```python
from build123d import *

# Parameters (mm, degrees)
BASE_DEPTH              = 5
BASE_DEPTH_BACK         = 5
ESQUISSE1_R             = 2
ESQUISSE2_W             = 77.5
ESQUISSE2_H             = 5
BOSS_EXTRU_2_DEPTH      = 10
ESQUISSE3_W             = 77.5
ESQUISSE3_H             = 5
BOSS_EXTRU_3_DEPTH      = 10
ESQUISSE4_W             = 5
ESQUISSE4_H             = 15
BOSS_EXTRU_4_DEPTH      = 5
ESQUISSE5_W             = 5
ESQUISSE5_H             = 15
ENL_V_MAT_EXTRU_1_DEPTH = 5


with BuildPart() as part:
    # Esquisse1 → BASE (new, two sides: drawn at the far end of the back side and taken through both)
    with BuildSketch(Plane.XY.offset(-BASE_DEPTH_BACK)):
        with BuildLine():
            Line((-80, 2.5), (0, 2.5))
            Line((0, 2.5), (0, -2.5))
            Line((0, -2.5), (-80, -2.5))
            ThreePointArc((-80, -2.5), (-82.5, 0), (-80, 2.5))
        make_face()
        with Locations((-80, 0)):
            Circle(ESQUISSE1_R, mode=Mode.SUBTRACT)
    extrude(amount=BASE_DEPTH + BASE_DEPTH_BACK)

    # Esquisse2 → Boss.-Extru.2 (add)
    with BuildSketch(Plane.XY.offset(5)):
        with Locations((-38.75, 0)):
            Rectangle(ESQUISSE2_W, ESQUISSE2_H)
    extrude(amount=BOSS_EXTRU_2_DEPTH)

    # Esquisse3 → Boss.-Extru.3 (add)
    with BuildSketch(Plane(origin=(0, 0, -5), x_dir=(-1, 0, 0), z_dir=(0, 0, -1))):
        with Locations((38.75, 0)):
            Rectangle(ESQUISSE3_W, ESQUISSE3_H)
    extrude(amount=BOSS_EXTRU_3_DEPTH)

    # Esquisse4 → Boss.-Extru.4 (add)
    with BuildSketch(Plane(origin=(0, 2.5, 0), x_dir=(1, 0, 0), z_dir=(0, 1, 0))):
        with Locations((2.5, 7.5)):
            Rectangle(ESQUISSE4_W, ESQUISSE4_H)
    extrude(amount=-BOSS_EXTRU_4_DEPTH)

    # Esquisse5 → Enlèv. mat.-Extru.1 (cut)
    with BuildSketch(Plane(origin=(0, 2.5, 0), x_dir=(1, 0, 0), z_dir=(0, 1, 0))):
        with Locations((-2.5, -7.5)):
            Rectangle(ESQUISSE5_W, ESQUISSE5_H)
    extrude(amount=-ENL_V_MAT_EXTRU_1_DEPTH, mode=Mode.SUBTRACT)


solid = part.part
```
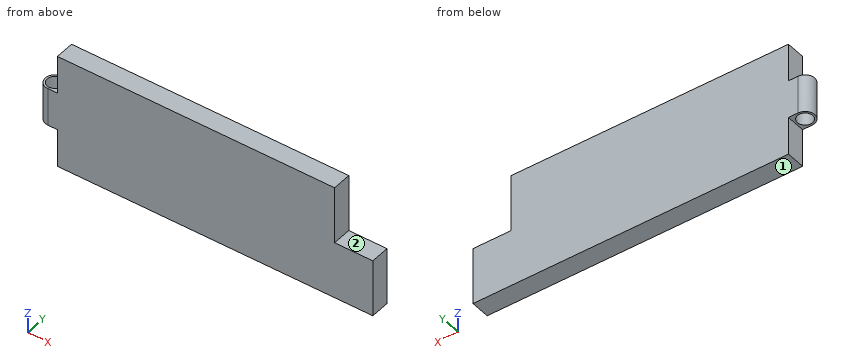
Could you check a few things on this model? Use its own coordinates, in mm. Face numbers are marked on the shaded views. A direction names the side the tool comes from. Coordinates: 2 decimals unless noted, no trailing zeros. Write each loop counter-clockwise with the first axis right and the second up, starting at its lowest first coordinate (ties: lowest second). Pieces come first, ordered by that corner, then holes. Notation, with made-up numbers: M 53,58 L 111,58 A22 cw 111,85 Z; hole C -14.5,-9 d4. An arc over 180 degrees is marked long. Answer as CSV lines item,"result". Start each with the question number.
1) I want a section at D-D, the plane z = 3.25. Please give me the cut outline in (x, y).
2) Please list where these lines run through material, in increasing order: line 1 (Y direction, x = -80, z = -2); line 2 (X direction, y = 0, z = -11); line 3 (Z direction, x = -1, y = 0.2). Write a range as from..to.
3) I want a section at B-B, the plane z = -1. Please give me the cut outline in (x, y).
4) For the marked faces 1 and 2, which set-ups out of +Z, -Z, +X, -X, +Y, -Y let a thin tool reach every point of the face, with its end or its side?
5) I want a section at A-A, the plane y = 0. Please give me the cut outline in (x, z).
6) For P1, Ø2.5, axis at x = -79.5, y = 0, coming from the +Z side; P2, Ø2.5, axis at y = 0.5, z = 6, coming from the +X side, each with a flat end and sliding along its axis, tell me the tip position at first contact or that it passes through.
7) I want a section at C-C, the plane z = 12.75. Please give me the cut outline in (x, y), and give its area (4 significant figures).
Data:
1,outline,"M -80,-2.5 L -5,-2.5 L -5,2.5 L -80,2.5 A2.5 ccw Z; hole C -80,0 d4"
2,line 1,"y = -2.5..-2, 2..2.5"
2,line 2,"x = -77.5..5"
2,line 3,"z = -15..0"
3,outline,"M -80,-2.5 L 5,-2.5 L 5,2.5 L -80,2.5 A2.5 ccw Z; hole C -80,0 d4"
4,face 1,"-Z, +X, -X, +Y, -Y"
4,face 2,"+Z, +X, +Y, -Y"
5,outline,"M -82.5,-5 L -82,-5 L -82,5 L -82.5,5 Z; M -78,-5 L -77.5,-5 L -77.5,-15 L 5,-15 L 5,0 L -5,0 L -5,15 L -77.5,15 L -77.5,5 L -78,5 Z"
6,P1,"passes through"
6,P2,"stops at x = -5"
7,outline,"M -77.5,-2.5 L -5,-2.5 L -5,2.5 L -77.5,2.5 Z"
7,area,"362.5 mm^2"
